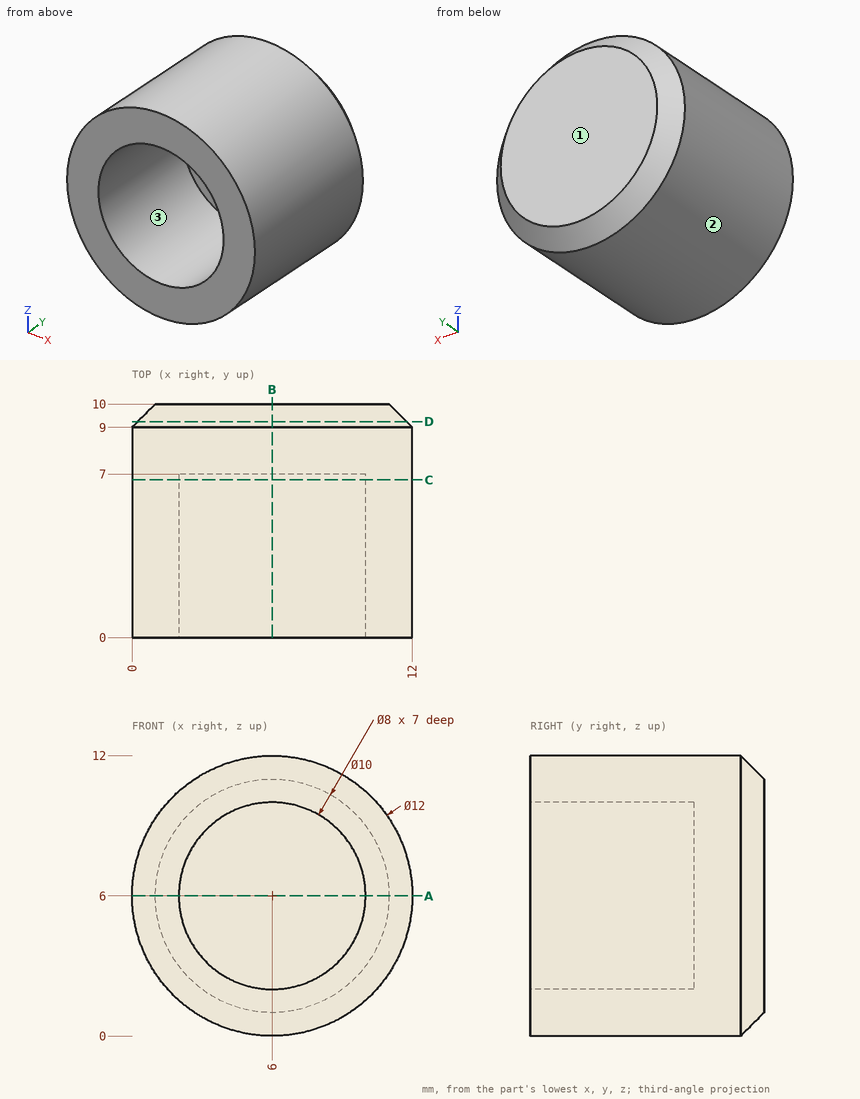
Source: three-view drawing plus pictorial views. Frame: mm from the lowest corner of the part. Give positions to 0.01 mm unless a question says otherwise; leave off trailing zeros. Order: outer loops, then holes, each group sorted by start corner. A loop starts at its lowest first (then second) coordinate and runs counter-clockwise, first axis right, second up. Notation, with made-up numbers: (-5, -19.75) -> (33, -19.75) arc R20 cw to (33, 3.25) -> close; hole circle Ø8 at (80.5, -23). An arc over 180 degrees is marked (long way). Put each result on its own line as item: value.
Q1. Section C-C, the plane y = 6.75. Return loops of the section in (x, z), then the cut area to 3 significant figures.
Here are the results:
outline: circle Ø12 at (6, 6); hole circle Ø8 at (6, 6)
area: 62.8 mm^2
Q2. Section D-D, the plane y = 9.25. Return loops of the section in (x, z).
Here are the results:
outline: circle Ø11.5 at (6, 6)
Q3. Pin query (flat end, axial travel): pin 1 (6 mm diameter, centred on x = 9.5, y = 5.5, fed in from -Z); pin 2 (5 mm diameter, centred on y = 8.5, z = 10, fed in from +X); pin 3 (7 mm diameter, centred on x = 6, z = 6, fed in from -Y). Return the tip coordinate at first contact, or that it passes through.
Here are the results:
pin 1: stops at z = 0.02
pin 2: stops at x = 11.81
pin 3: stops at y = 7
Q4. Material intervals for L1, parallel to Z at x = 6, y = 3.5; L2, parallel to Y at x = 7.25, z = 4.5; L3, parallel to Z at x = 9.25, y = 4.75, sorted ascending.
Here are the results:
L1: z = 0 to 2, 10 to 12
L2: y = 7 to 10
L3: z = 0.96 to 3.67, 8.33 to 11.04
Q5. Section B-B, the plane x = 6. Return loops of the section in (y, z).
Here are the results:
outline: (0, 0) -> (9, 0) -> (10, 1) -> (10, 11) -> (9, 12) -> (0, 12) -> (0, 10) -> (7, 10) -> (7, 2) -> (0, 2) -> close
Q6. Draft query along Z for the marked faces 1, 2 and 3. Return one class per face: released by +Z, released by -Z, zero draft, split by the parting line, or undercut.
Here are the results:
face 1: zero draft
face 2: split by the parting line
face 3: undercut
Q7. Section A-A, the plane z = 6. Return loops of the section in (x, y), then the cut area to 3 significant figures.
Here are the results:
outline: (0, 0) -> (2, 0) -> (2, 7) -> (10, 7) -> (10, 0) -> (12, 0) -> (12, 9) -> (11, 10) -> (1, 10) -> (0, 9) -> close
area: 63.0 mm^2
